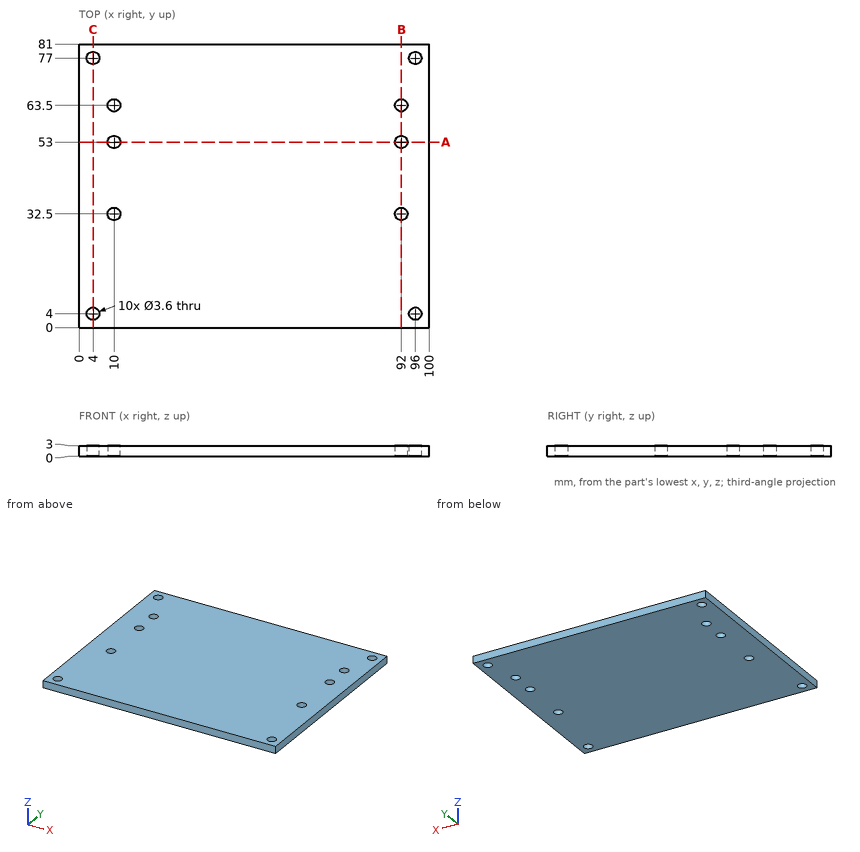
Study the drawing (mm; zero at the part's minimum x, y, z) and answer. Coordinates: 2 decimals unless noted, no trailing zeros. Loops run counter-clockwise (first coordinate to the right, second up) from the corner with the lowest first, then second, coordinate; pieces in that order, holes last. Notation, with made-up numbers: M 7,51 L 16,51 A7 ccw 16,64 Z; hole C 36,-9 d9. An arc over 180 degrees is marked long. Answer in a Markdown table with one row per item. Add a question column.
1. Find section B-B, the plane x = 92. Write down the section's boundary in (y, z), then the cut area to 3 significant figures.
2. Find section C-C, the plane x = 4. Write down the section's boundary in (y, z).
3. Consider L1, parallel to X at y = 63.5, z = 0.95; L2, parallel to Y at x = 96, z = 1; L3, parallel to Y at x = 92, z = 1.6. Determine where each line is inside the solid, lowest interval first.
4. Flat-ended cylindrical pins translate along their axes: P1, Ø1.5, axis at y = 58.5, z = 0.5, coming from the -X side; P2, Ø3, axis at x = 96, y = 4, coming from the +Z side. Find the tip coordinate at first contact, or state that the pin passes through.
5. Find section A-A, the plane y = 53. Write down the section's boundary in (x, z).
Reported:
| question | item | result |
|---|---|---|
| 1 | outline | M 0,0 L 30.7,0 L 30.7,3 L 0,3 Z; M 34.3,0 L 51.2,0 L 51.2,3 L 34.3,3 Z; M 54.8,0 L 61.7,0 L 61.7,3 L 54.8,3 Z; M 65.3,0 L 81,0 L 81,3 L 65.3,3 Z |
| 1 | area | 211 mm^2 |
| 2 | outline | M 0,0 L 2.2,0 L 2.2,3 L 0,3 Z; M 5.8,0 L 75.2,0 L 75.2,3 L 5.8,3 Z; M 78.8,0 L 81,0 L 81,3 L 78.8,3 Z |
| 3 | L1 | x = 0 to 8.2, 11.8 to 90.2, 93.8 to 100 |
| 3 | L2 | y = 0 to 2.2, 5.8 to 75.2, 78.8 to 81 |
| 3 | L3 | y = 0 to 30.7, 34.3 to 51.2, 54.8 to 61.7, 65.3 to 81 |
| 4 | P1 | stops at x = 0 |
| 4 | P2 | passes through |
| 5 | outline | M 0,0 L 8.2,0 L 8.2,3 L 0,3 Z; M 11.8,0 L 90.2,0 L 90.2,3 L 11.8,3 Z; M 93.8,0 L 100,0 L 100,3 L 93.8,3 Z |
